Read the model definition and answer for the solid it produces. Units are mm, in the model's axes. Face numbers are marked on the shaded views. Give positions to 0.01 mm unless a question says otherwise; leave off trailing zeros. Loops run counter-clockwise (first coordinate to the right, second up) from the corner with the lowest first, then second, coordinate; pieces in that order, holes last. Notation, with made-up numbers: (-3, -4) - (38, -4) arc R28 cw to (38, 33) - close; hole circle Ø2 at (8.5, 14). An arc over 180 degrees is marked (long way). Write item = value, one per line.
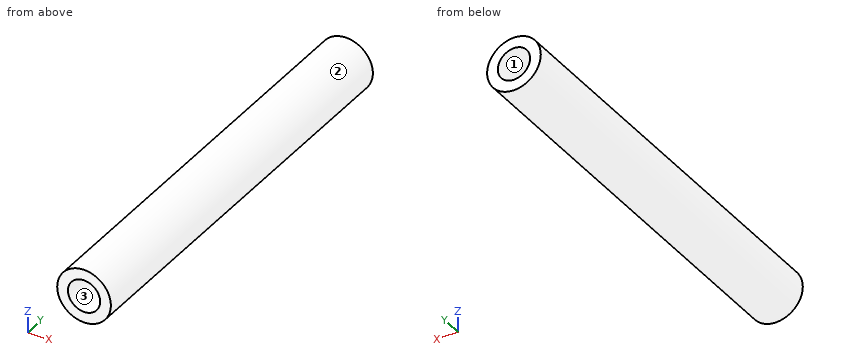
Autodesk Inventor part; units mm, degrees
ref_plane "YZ Plane" through (0, 0, 0) normal (1, 0, 0) x (0, 1, 0)
ref_plane "XZ Plane" through (0, 0, 0) normal (0, 1, 0) x (-1, 0, 0)
ref_plane "XY Plane" through (0, 0, 0) normal (0, 0, 1) x (1, 0, 0)
sketch "Sketch1" plane through (0, 0, 0) normal (0, 1, 0) x (-1, 0, 0)
  circle A0 centre (0, 0) radius 1.1906
  circle A1 centre (0, 0) radius 0.715
  dimension "d0" = 2.3813
  dimension "d1" = 1.43
extrude "Extrusion1" add sketch "Sketch1" along normal blind 9.271 contours A0 | A1
extrude "Extrusion2" cut sketch "Sketch1" along normal blind 6.35 contours A1
mirror "Mirror1" about plane through (0, 9.271, 0) normal (0, 1, 0)
properties part number "Frame Post"
1) A cutting plane is placed at A-A on z = 0. Determine the outline of the cut face in (x, y) (3 decimals).
Output:
outline = (-1.191, 0) - (-0.715, 0) - (-0.715, 6.35) - (0.715, 6.35) - (0.715, 0) - (1.191, 0) - (1.191, 18.542) - (0.715, 18.542) - (0.715, 12.192) - (-0.715, 12.192) - (-0.715, 18.542) - (-1.191, 18.542) - close
2) A cutting plane is placed at D-D on z = 1. Determine the outline of the cut face in (x, y), then the cut area to 3 significant figures.
Output:
outline = (-0.65, 0) - (0.65, 0) - (0.65, 18.54) - (-0.65, 18.54) - close
area = 24.0 mm²
3) Find the intervals of material crossed by probe 1 along Z at (x, y) = (0, 3) (3 decimals); probe 2 along Y at (x, z) = (-0.35, 0.35); probe 3 along X at (y, z) = (13, 0.15), in increasing order.
Output:
probe_1 = -1.191 to -0.715, 0.715 to 1.191
probe_2 = 6.35 to 12.19
probe_3 = -1.18 to -0.7, 0.7 to 1.18
4) A cutting plane is placed at C-C on y = 13.5. Determine the outline of the cut face in (x, z) (3 decimals).
Output:
outline = circle Ø2.381 at (0, 0); hole circle Ø1.43 at (0, 0)
5) This flat-tipped pin is pushed along its axis until it touches: P1, Ø1.1, axis at x = 0, z = 0, coming from the -Y side. Where does it stop, or does it pass through?
Output:
P1 = 6.35
6) The mould has two halves that part along Z. Classify the marked faces 1, 2 and 3: pulls with the +Z half, pulls with the -Z half, needs draft (parallel to the pull), parting line crosses it, or undercut.
Output:
face_1 = undercut
face_2 = parting line crosses it
face_3 = undercut
7) A cutting plane is placed at B-B on x = 0. Determine the outline of the cut face in (y, z) (3 decimals), then the cut area to 3 significant figures.
Output:
outline = (0, -1.191) - (18.542, -1.191) - (18.542, -0.715) - (12.192, -0.715) - (12.192, 0.715) - (18.542, 0.715) - (18.542, 1.191) - (0, 1.191) - (0, 0.715) - (6.35, 0.715) - (6.35, -0.715) - (0, -0.715) - close
area = 26.0 mm²
